The listing builds one solid part. Answer for the finished solid, in the listing's coordinates (mm). Coordinates: 2 decimals unless noted, no trailing zeros. Order: outer loops, then holes, each group sorted by start corner. A loop starts at its lowest first (then second) coordinate and runs counter-clockwise, first axis right, second up. Notation, with made-up numbers: (32.5, 79.25) - (91.5, 79.25) arc R18 cw to (91.5, 110.25) - close; hole circle Ø6 at (-25.5, 44.25). An arc over 180 degrees is marked (long way). Use one line per item in the form item = value. Start each with the question number.
Item 1: Section A-A, the plane x = 348 is taken. Write down the section's boundary in (y, z).
Item 2: Consider line 1 along Z through (x, y) = (-401.25, -6.35); line 2 along Y through (x, z) = (393, 25.4); line 3 along Z through (x, y) = (-210, -8). Determine where each line is inside the solid, lowest interval first. Write a range as [from, to].
Item 3: Each of these flat-tipped pins is pushed along its axis until it touches: pin 1 Ø6.5 at (y, z) = (-6.35, 25.4) entering from -X; pin 2 Ø5 at (y, z) = (-6.35, 25.4) entering from +X; pin 3 Ø6.5 at (y, z) = (-6.35, -12.7) entering from +X. Where does it stop, or does it pass through?
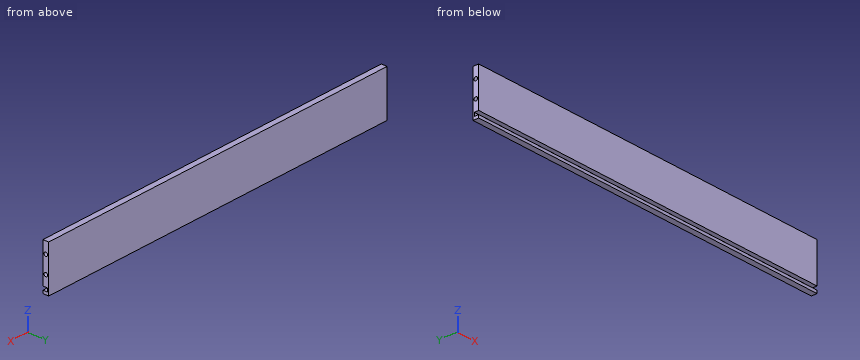
from build123d import *

# Parameters (mm, degrees)
F0_W     = 823.976
F0_H     = 101.6
F1_DEPTH = 12.7
F2_W     = 823.976
F2_H     = 7.874
F3_DEPTH = 9.652
F5_D     = 8.001
F5_DEPTH = 25.4
F5_TIP   = 2.4037429064
F7_D     = 8.001
F7_DEPTH = 25.4
F7_TIP   = 2.4037429064


# Not quite as in the source:
# - a feature names something its author has since deleted; it is built from what else it names


with BuildPart() as f1:
    # F0 (on Front) → F1 (new body)
    with BuildSketch(Plane.XZ):
        Rectangle(F0_W, F0_H)
    extrude(amount=F1_DEPTH)

    # F2 (on face) → F3 (cut)
    with BuildSketch(Plane.XZ.offset(12.7)):
        with Locations((0, -40.513)):
            Rectangle(F2_W, F2_H)
    extrude(amount=-F3_DEPTH, mode=Mode.SUBTRACT)

    # F5
    with Locations(Plane(origin=(-411.988, 0, 0), x_dir=(0, -1, 0), z_dir=(-1, 0, 0))):
        with Locations((6.35, 25.4), (6.35, -12.7)):
            Hole(F5_D / 2, depth=F5_DEPTH)
            with Locations((0, 0, -(F5_DEPTH + F5_TIP / 2))):  # 118° drill point
                Cone(0, F5_D / 2, F5_TIP, mode=Mode.SUBTRACT)

    # F7
    with Locations(Plane.YZ.offset(411.988)):
        with Locations((-6.35, 25.4), (-6.35, -12.7)):
            Hole(F7_D / 2, depth=F7_DEPTH)
            with Locations((0, 0, -(F7_DEPTH + F7_TIP / 2))):  # 118° drill point
                Cone(0, F7_D / 2, F7_TIP, mode=Mode.SUBTRACT)


solid = f1.part
Response:
q1.outline = (-12.7, -50.8) - (0, -50.8) - (0, 50.8) - (-12.7, 50.8) - (-12.7, -36.58) - (-3.05, -36.58) - (-3.05, -44.45) - (-12.7, -44.45) - close
q2.line_1 = [-50.8, -44.45], [-36.58, -16.7], [-8.7, 21.4], [29.4, 50.8]
q2.line_2 = [-12.7, -10.35], [-2.35, 0]
q2.line_3 = [-50.8, -44.45], [-36.58, 50.8]
q3.pin_1 = -386.14
q3.pin_2 = 385.69
q3.pin_3 = 386.14
